Work out the finished part from the listing and answer in its coordinate system (mm). Coordinates: 2 decimals unless noted, no trailing zeros. Write each question's results on one line, items separated by ' | '. Start each with the question number.
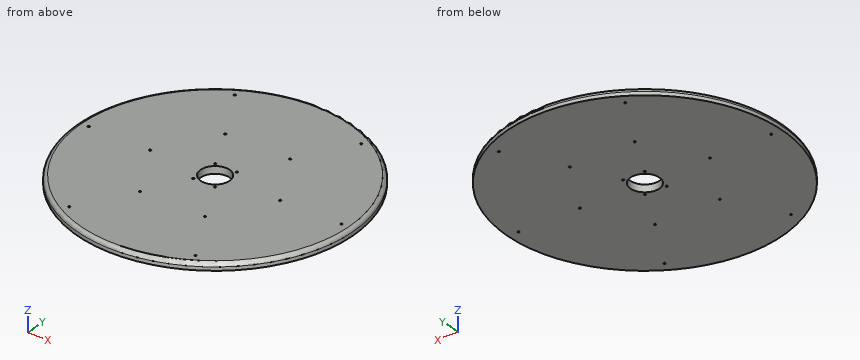
from build123d import *

# Parameters (mm, degrees)
F0_R     = 241.3
F0_R_2   = 1.7272
F0_R_3   = 25.4
F1_DEPTH = 12.7
F2_R     = 1.7272
F3_DEPTH = 12.7
F4_R     = 6.35


with BuildPart() as f1:
    # F0 (on Top) → F1 (new body)
    with BuildSketch(Plane.XY):
        Circle(F0_R)
        with Locations((-111.125, -192.474146)):
            Circle(F0_R_2, mode=Mode.SUBTRACT)
        with Locations((111.125, -192.474146)):
            Circle(F0_R_2, mode=Mode.SUBTRACT)
        with Locations((-222.25, 0)):
            Circle(F0_R_2, mode=Mode.SUBTRACT)
        with Locations((-111.125, 192.474146)):
            Circle(F0_R_2, mode=Mode.SUBTRACT)
        Circle(F0_R_3, mode=Mode.SUBTRACT)
        with Locations((222.25, 0)):
            Circle(F0_R_2, mode=Mode.SUBTRACT)
        with Locations((111.125, 192.474146)):
            Circle(F0_R_2, mode=Mode.SUBTRACT)
    extrude(amount=F1_DEPTH)

    # F2 (on face) → F3 (cut, through all)
    with BuildSketch(Plane.XY.offset(12.7)):
        with Locations((-57.15, 98.986704)):
            Circle(F2_R)
        with Locations((57.15, 98.986704)):
            Circle(F2_R)
        with Locations((-114.3, 0)):
            Circle(F2_R)
        with Locations((-57.15, -98.986704)):
            Circle(F2_R)
        with Locations((57.15, -98.986704)):
            Circle(F2_R)
        with Locations((114.3, 0)):
            Circle(F2_R)
        with Locations((-19.05, -25.4)):
            Circle(F2_R)
        with Locations((19.05, -25.4)):
            Circle(F2_R)
        with Locations((19.05, 25.4)):
            Circle(F2_R)
        with Locations((-19.05, 25.4)):
            Circle(F2_R)
    extrude(amount=-F3_DEPTH, mode=Mode.SUBTRACT)

    # F4
    f4_edges = [f1.edges().sort_by_distance(p)[0] for p in [
        (-241.3, 0, 12.7),
    ]]
    fillet(f4_edges, radius=F4_R)


solid = f1.part
1. Given pin 1 Ø5.5 at (x, y) = (19.05, 25.4) entering from +Z; pin 2 Ø3 at (x, y) = (-111.12, 192.47) entering from -Z; pin 3 Ø1.5 at (x, z) = (97.5, 10.5) entering from -Y; pin 4 Ø4 at (y, z) = (80, 5.5) entering from -X, each flat-ended and moving along its own axis, determine where each tip first touches the part or whether it passes through.
2. Find section A-A on z = 9. Give the number of separate pieces and of enclosed holes in the cut face, and give its area (3 significant figures).
3. Find the intervals of material crossed by L1, parallel to Y at x = -57.15, z = 4.75; L2, parallel to Y at x = 222.25, z = 3.5; L3, parallel to Y at x = 57.15, z = 8.5, in increasing order.
Ans:
1) pin 1: stops at z = 12.7 | pin 2: passes through | pin 3: stops at y = -219.74 | pin 4: stops at x = -228.35
2) separate pieces: 1 | enclosed holes: 17 | area: 180,000 mm²
3) L1: y = -234.43 to -100.71, -97.26 to 97.26, 100.71 to 234.43 | L2: y = -93.97 to -1.73, 1.73 to 93.97 | L3: y = -234.05 to -100.71, -97.26 to 97.26, 100.71 to 234.05
